Study the drawing (mm; zero at the part's minimum x, y, z) and answer. A direction names the side the tool comes from. Round coordinates to 2 decimals unless told otherwise and drop trailing zeros. Loops run counter-clockwise (first coordinate to the right, second up) from the corner with the lowest first, then second, coordinate; pieces in that order, holes last. Notation, with made-up numbers: M -32.5,54.5 L 11.5,54.5 A20 cw 11.5,81.5 Z; hole C 21.5,81 d10. An arc over 180 degrees is marked long. Put each result on its own line as item: value. Start each with the question number.
(1) Section D-D, the plane x = 44 is taken. Determine the outline of the cut face in (y, z), then the cut area to 3 significant figures.
(2) Section B-B, the plane x = 20 is taken. Determine the outline of the cut face in (y, z).
(3) Flat-ended cylindrical pins translate along their axes: P1, Ø5, axis at y = 13.5, z = 3, coming from the +X side; P2, Ø3.5, axis at x = 30, z = 5, coming from the +Y side. Find the tip coordinate at first contact, or state that the pin passes through.
(4) Which of the six approach directions +Z, -Z, +X, -X, +Y, -Y give full straight-line access (tool end or side, diameter ignored) to the marked faces 5, 6 and 7?
(5) Section C-C, the plane z = 12.5 is taken. Determine the outline of the cut face in (x, y), then the cut area to 3 significant figures.
(6) Straight lines are drawn through the part: line 1 (Z direction, x = 30, y = 4.05); line 2 (X direction, y = 12, z = 2); line 3 (X direction, y = 1.25, z = 7.5). For each, find the intervals that lie inside material, in ascending order.
(7) Determine the mould class of the marked faces 1, 2, 3 and 4 for opening direction X: released by +X, released by -X, zero draft, split by the parting line, or undercut.
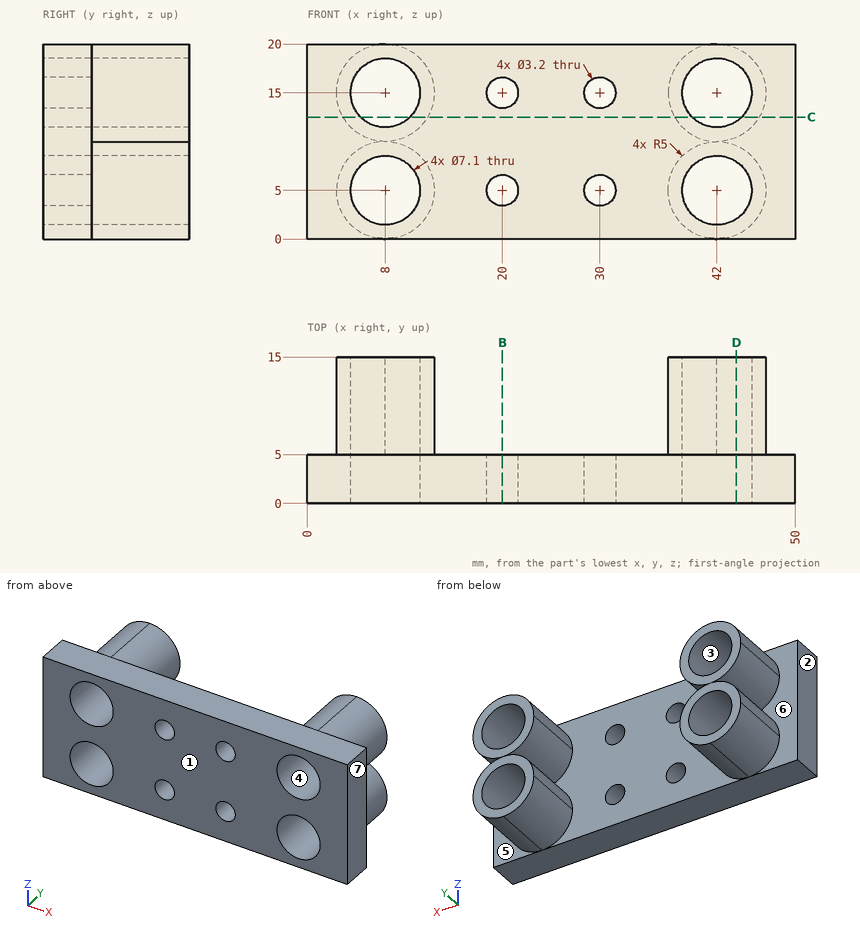
Recorded:
1. outline: M 0,0 L 5,0 L 5,0.42 L 15,0.42 L 15,2.07 L 0,2.07 Z; M 0,7.93 L 15,7.93 L 15,9.58 L 5,9.58 L 5,10.42 L 15,10.42 L 15,12.07 L 0,12.07 Z; M 0,17.93 L 15,17.93 L 15,19.58 L 5,19.58 L 5,20 L 0,20 Z
1. area: 107 mm²
2. outline: M 0,0 L 5,0 L 5,3.4 L 0,3.4 Z; M 0,6.6 L 5,6.6 L 5,13.4 L 0,13.4 Z; M 0,16.6 L 5,16.6 L 5,20 L 0,20 Z
3. P1: stops at x = 47
3. P2: stops at y = 5
4. face 5: +X, +Y
4. face 6: -X, +Y
4. face 7: +Z, -Z, +X, +Y, -Y
5. outline: M 0,0 L 5.48,0 L 5.48,15 L 3.67,15 L 3.67,5 L 0,5 Z; M 10.52,0 L 39.48,0 L 39.48,15 L 37.67,15 L 37.67,5 L 12.33,5 L 12.33,15 L 10.52,15 Z; M 44.52,0 L 50,0 L 50,5 L 46.33,5 L 46.33,15 L 44.52,15 Z
5. area: 272 mm²
6. line 1: z = 0 to 3.4, 6.6 to 13.4, 16.6 to 20
6. line 2: x = 4 to 6.1, 9.9 to 12, 38 to 40.1, 43.9 to 46
6. line 3: x = 0 to 5.48, 10.52 to 39.48, 44.52 to 50
7. face 1: zero draft
7. face 2: released by -X
7. face 3: undercut
7. face 4: undercut
